Autodesk Inventor part; units mm, degrees
ref_plane "YZ Plane" through (0, 0, 0) normal (1, 0, 0) x (0, 1, 0)
ref_plane "XZ Plane" through (0, 0, 0) normal (0, 1, 0) x (-1, 0, 0)
ref_plane "XY Plane" through (0, 0, 0) normal (0, 0, 1) x (1, 0, 0)
sketch "スケッチ1" plane through (0, 0, 0) normal (0, 0, 1) x (1, 0, 0)
  line L0 (-15.75, 60) -> (15.75, 60)
  line L1 (15.75, 60) -> (15.75, -60)
  line L2 (15.75, -60) -> (-15.75, -60)
  line L3 (-15.75, -60) -> (-15.75, 60)
  point P0 (0, 0)
  dimension "d0" = 31.5
  dimension "d1" = 15.75
  dimension "d2" = 120
  dimension "d3" = 60
extrude "押し出し1" add sketch "スケッチ1" along normal blind 4
fillet "フィレット1" radius 15.75 4 edges at (-15.75, -60, 2) (15.75, -60, 2) (15.75, 60, 2) (-15.75, 60, 2)
sketch "スケッチ2" plane through (0, 0, 4) normal (0, 0, 1) x (1, 0, 0)
  arc A0 (15.75, 44.25) -> (-15.75, 44.25) centre (0, 44.25) ccw
  circle A1 centre (0, 44.25) radius 14
  point P0 (0, 0)
  dimension "d7" = 28
extrude "押し出し2" cut sketch "スケッチ2" against normal through all
sketch "スケッチ3" plane through (0, 0, 4) normal (0, 0, 1) x (1, 0, 0)
  arc A0 (15.75, 44.25) -> (-15.75, 44.25) centre (0, 44.25) ccw
  circle A1 centre (0, 44.25) radius 19.5
  line L0 (0, 44.25) -> (0, 24.75)
  line L1 (0, 44.25) -> (9.75, 27.3625)
  line L2 (0, 44.25) -> (-9.75, 27.3625)
  line L3 (0, 44.25) -> (0, 63.75)
  point P0 (0, 0)
  point P1 (9.75, 27.3625)
  dimension "d10" = 39
  dimension "d11" = 150
  dimension "d13" = 30
hole "Hole1" at (-9.75, 27.3625, 4) at (9.75, 27.3625, 4) at (0, 24.75, 4) direction (0, 0, -1) diameter 3.2 depth 8 tip angle 118
sketch "スケッチ4" plane through (0, 0, 4) normal (0, 0, 1) x (1, 0, 0)
  arc A0 (-15.75, -44.25) -> (15.75, -44.25) centre (0, -44.25) ccw
  point P0 (0, 0)
hole "Hole2" at (0, -44.25, 4) direction (0, 0, -1) diameter 4 end through all counterbore diameter 12.5 counterbore depth 0.8
sketch "スケッチ5" plane through (0, 0, 4) normal (0, 0, 1) x (1, 0, 0)
  circle A0 centre (0, -44.25) radius 13.25
  circle A1 centre (0, -44.25) radius 9.25
  point P0 (0, 0)
  dimension "d28" = 26.5
  dimension "d29" = 18.5
extrude "押し出し3" cut sketch "スケッチ5" against normal blind 3
equation "\"d6\" = 0.5 * d0"
properties part number "JointC3'B_2nd" material "アルミニウム 6061"
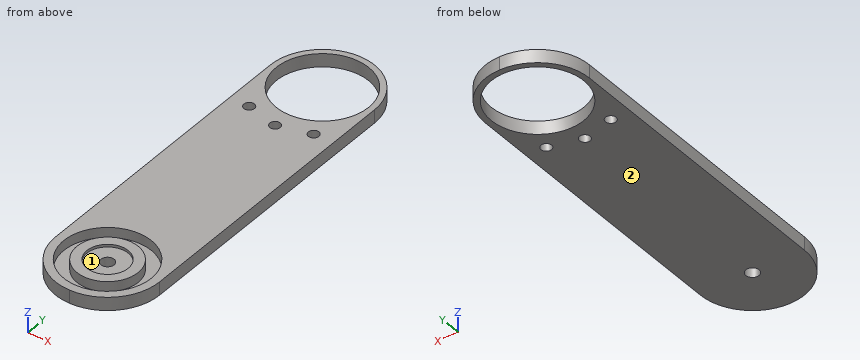
Check sheet for the modelled part. Datum: model origin and axes. Units: mm. Face numbers are marked on the shaded views. Give positions to 0.01 mm unless a question says otherwise; leave off trailing zeros. Loops run counter-clockwise (first coordinate to the right, second up) from the corner with the lowest first, then second, coordinate; pieces in that order, holes last. Notation, with made-up numbers: M 69.25,-3.75 L 80.25,-3.75 A22 cw 80.25,13.25 Z; hole C 45.5,43 d8. An arc over 180 degrees is marked long. Answer as a JSON object with one key per item and string values. Group by question number.
Q1. Cross-section at D-D on x = -4.5. Record the cut outline in (y, z).
Q2. Go/stop test with flat-tipped pins: P1, Ø1, axis at x = -11.5, z = 3.5, coming from the +Y side; P2, Ø6, axis at x = 2.5, y = -43.5, coming from the +Z side. Record where each tip stops, or that it passes through.
Q3. Cross-section at A-A on z = 2.25. Give the number of separate pieces and of enclosed holes in the cut face, then the cut area to 3 significant figures.
Q4. Cross-section at B-B on y = 46. Record the cut outline in (x, z), then the cut area to 3 significant figures.
Q5. Release check for a two-part mould opening along X. For the marked faces 1 and 2 record: released by +X, released by -X, zero draft, split by the parting line, or undercut.
Q6. Cross-section at C-C on x = 4. Record the cut outline in (y, z).
Q7. Material ranges on line 1 along Y through (x, z) = (0, 1.75); line 2 along X through (y, z) = (-36, 3); line 3 along Y through (x, z) = (-5, 1.6), recorded low to high. Write a range as [from, to].
Evaluation:
{
 "1": {"outline": "M -59.34,0 L 30.99,0 L 30.99,4 L -31.79,4 L -31.79,1 L -36.17,1 L -36.17,4 L -39.91,4 L -39.91,3.2 L -48.59,3.2 L -48.59,4 L -52.33,4 L -52.33,1 L -56.71,1 L -56.71,4 L -59.34,4 Z; M 57.51,0 L 59.34,0 L 59.34,4 L 57.51,4 Z"},
 "2": {"P1": "stops at y = 55.52", "P2": "stops at z = 3.2"},
 "3": {"separate pieces": "2", "enclosed holes": "6", "area": "2,630 mm2"},
 "4": {"outline": "M -15.65,0 L -13.89,0 L -13.89,4 L -15.65,4 Z; M 13.89,0 L 15.65,0 L 15.65,4 L 13.89,4 Z", "area": "14.1 mm2"},
 "5": {"face 1": "undercut", "face 2": "zero draft"},
 "6": {"outline": "M -59.48,0 L 30.83,0 L 30.83,4 L -31.62,4 L -31.62,1 L -35.91,1 L -35.91,4 L -39.45,4 L -39.45,3.2 L -49.05,3.2 L -49.05,4 L -52.59,4 L -52.59,1 L -56.88,1 L -56.88,4 L -59.48,4 Z; M 57.67,0 L 59.48,0 L 59.48,4 L 57.67,4 Z"},
 "7": {"line 1": "y = [-60, -57.5], [-53.5, -46.25], [-42.25, -35], [-31, 23.15], [26.35, 30.25], [58.25, 60]", "line 2": "x = [-15.75, -10.37], [-4.18, 4.18], [10.37, 15.75]", "line 3": "y = [-59.19, -56.52], [-52.03, -36.47], [-31.98, 31.17], [57.33, 59.19]"}
}
